Part model, mm, in its own coordinate system. Face numbers are marked on the shaded views. A direction names the side the tool comes from. Give positions to 0.01 mm unless a question says otherwise; leave off trailing zeros. Order: outer loops, then holes, each group sorted by start corner. A loop starts at its lowest first (then second) coordinate and runs counter-clockwise, first axis right, second up.
1. Slice it at B-B on y = -17. List the corners of the cut face in (x, z), and give its area (3 significant figures).
2. Slice it at D-D on x = 7.5. List the corners of the cut face in (y, z), and give its area (3 significant figures).
3. Which spindle directions (+Z, -Z, +X, -X, +Y, -Y) get a long thin tool onto all of the face, cutting with end or side? Do the marked faces 4, 5 and 6. Say none if no direction does.
4. Slice it at C-C on z = 8.5. List the corners of the cut face in (x, y), and give its area (3 significant figures).
5. Probe line 1 (Z direction, x = 50, y = 10); line 2 (X direction, y = 9.5, z = 26.5); line 3 (Y direction, x = 40, z = 8.5). List the from-to ranges inside material, lowest first.
6. Drop flat-ended pins along their axis: pin 1 Ø1 at (x, y) = (43.5, 2.5) entering from +Z; pin 2 Ø6 at (y, z) = (16, 38.5) entering from -X; pin 3 Ø3.5 at (x, z) = (51, 4) entering from +Y; pin 4 Ø20.5 at (x, y) = (-18.31, 0.77) entering from -Z. Give the stop position or say it passes through.
7. Slice it at A-A on x = 61. List the corners of the cut face in (y, z).
8. Mould opens along X. For the marked faces 1, 2 and 3 say: +X half, -X half, draft (parallel to the pull), parting line (faces both ways), or undercut.
from build123d import *

# Parameters (mm, degrees)
F0_W     = 107.95
F0_H     = 50.8
F0_R     = 7.874
F1_DEPTH = 11.176
F3_DEPTH = 33.401
F4_DEPTH = 41.148
F5_DEPTH = 33.401
F6_W     = 41.148
F6_H     = 20.574
F7_DEPTH = 49.5820905122
F8_R     = 20.57399


# Not quite as in the source:
# - a fillet or chamfer is up to 0.001 mm smaller than in the source, because OpenCascade refuses the exact size


with BuildPart() as f1:
    # F0 (on Top) → F1 (new body)
    with BuildSketch(Plane.XY):
        with Locations((18.2708286419, 0.7708109915)):
            Rectangle(F0_W, F0_H)
        with Locations((-18.3051713581, 0.7708109915)):
            Circle(F0_R, mode=Mode.SUBTRACT)
        with Locations((54.8468286419, 0.7708109915)):
            Circle(F0_R, mode=Mode.SUBTRACT)
    extrude(amount=F1_DEPTH)



with BuildPart() as f3:
    # F2 (on face) → F3 (new body)
    with BuildSketch(Plane(origin=(-35.7041713581, 0, 0), x_dir=(0, -1, 0), z_dir=(-1, 0, 0))):
        Polygon((-26.1708109915, 11.176), (24.6291890085, 11.176), (6.3411890085, 42.8517451688), (-36.5981609479, 18.0606999127), (-26.1708109915, 0), align=None)
    extrude(amount=-F3_DEPTH)


with BuildPart() as f1_1:
    add(f1.part)
    # F4 (add): a face of the model
    f4_faces = [f3.part.faces().sort_by_distance(p)[0] for p in [
        (-2.3031713581, 4.9580328492, 21.6795412193),
    ]]

    add(f3.part)  # F4 merges F3
    extrude(f4_faces, amount=F4_DEPTH)

    # F2 (on face) → F5 (cut)
    with BuildSketch(Plane(origin=(-35.7041713581, 0, 0), x_dir=(0, -1, 0), z_dir=(-1, 0, 0))):
        Polygon((-26.1708109915, 11.176), (24.6291890085, 11.176), (6.3411890085, 42.8517451688), (-36.5981609479, 18.0606999127), (-26.1708109915, 0), align=None)
    extrude(amount=-F5_DEPTH, mode=Mode.SUBTRACT)

    # F6 (on face) → F7 (join, through all)
    with BuildSketch(Plane(origin=(0, -23.3112417127, 13.458751678), x_dir=(1, 0, 0), z_dir=(0, -0.8660254038, 0.5))):
        with Locations((18.2708286419, 44.2271054085)):
            Rectangle(F6_W, F6_H)
    extrude(amount=-F7_DEPTH)

    # F8 (radius 20.574 in the source; OpenCascade refuses exactly that, so slightly less here)
    f8_edges = [f1_1.edges().sort_by_distance(p)[0] for p in [
        (38.844829, 25.415486, 48.273829),
        (-2.303171, 25.415486, 48.273829),
    ]]
    fillet(f8_edges, radius=F8_R)


solid = f1_1.part
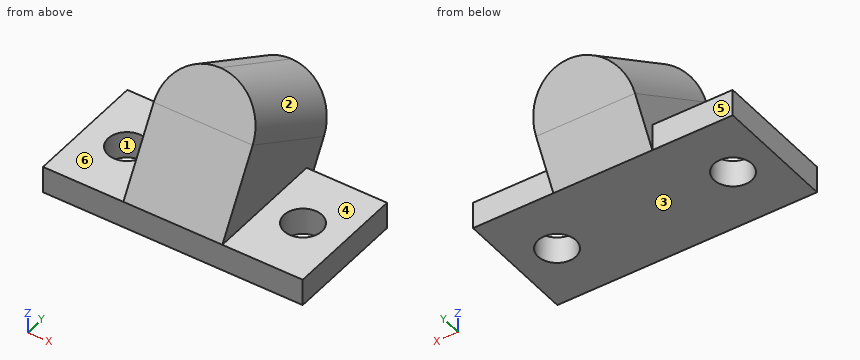
Data:
1. outline: (-35.7, 0) - (72.25, 0) - (72.25, 11.18) - (38.84, 11.18) - (38.84, 24.39) - (-2.3, 24.39) - (-2.3, 11.18) - (-35.7, 11.18) - close
1. area: 1,750 mm2
2. outline: (-24.63, 0) - (26.17, 0) - (45.36, 33.24) - (2.42, 58.03) - (-24.63, 11.18) - close
2. area: 2,580 mm2
3. face 4: +Z, +X, +Y, -Y
3. face 5: +Z, -Z, -X, +Y
3. face 6: +Z, -X, +Y, -Y
4. outline: (-35.7, -24.63) - (72.25, -24.63) - (72.25, 26.17) - (38.84, 26.17) - (38.84, 31.08) - (-2.3, 31.08) - (-2.3, 26.17) - (-35.7, 26.17) - close; hole circle Ø15.75 at (-18.31, 0.77); hole circle Ø15.75 at (54.85, 0.77)
4. area: 5,300 mm2
5. line 1: z = 0 to 11.18
5. line 2: x = -2.3 to 38.84
5. line 3: y = -24.63 to 26.17
6. pin 1: stops at z = 11.18
6. pin 2: stops at x = -1.83
6. pin 3: stops at y = 26.17
6. pin 4: stops at z = 0
7. outline: (-24.63, 0) - (-4.14, 0) - (-4.14, 11.18) - (-24.63, 11.18) - close; (5.68, 0) - (26.17, 0) - (26.17, 11.18) - (5.68, 11.18) - close
8. face 1: undercut
8. face 2: +X half
8. face 3: draft
